```python
from build123d import *

# Parameters (mm, degrees)
F0_R      = 5
F1_DEPTH  = 15
F2_R      = 5
F4_DEPTH  = 15
F3_R      = 2.6
F5_DEPTH  = 25
F6_R      = 1.5
F7_DEPTH  = 10
F8_R      = 3.1
F9_DEPTH  = 1.5
F10_R     = 1.425
F11_DEPTH = 25
F12_R     = 2
F13_DEPTH = 1.5


with BuildPart() as f1:
    # F0 (on Front) → F1 (new body)
    with BuildSketch(Plane.XZ):
        Circle(F0_R)
    extrude(amount=F1_DEPTH)

    # F2 (on Top) → F4 (join)
    with BuildSketch(Plane.XY):
        with Locations((0, -9.121813)):
            Circle(F2_R)
    extrude(amount=F4_DEPTH)

    # F3 (on Front) → F5 (cut)
    with BuildSketch(Plane.XZ):
        Circle(F3_R)
    extrude(amount=F5_DEPTH, mode=Mode.SUBTRACT)

    # F6 (on face) → F7 (cut)
    with BuildSketch(Plane.XY.offset(15)):
        with Locations((0, -9.121813)):
            Circle(F6_R)
    extrude(amount=-F7_DEPTH, mode=Mode.SUBTRACT)

    # F8 (on face) → F9 (cut)
    with BuildSketch(Plane.XY.offset(15)):
        with Locations((0, -9.121813)):
            Circle(F8_R)
    extrude(amount=-F9_DEPTH, mode=Mode.SUBTRACT)

    # F10 (on Right) → F11 (cut)
    with BuildSketch(Plane.YZ):
        with Locations((-8.868461, 9.550918)):
            Circle(F10_R)
    extrude(amount=F11_DEPTH, mode=Mode.SUBTRACT)

    # F12 (on face) → F13 (cut)
    with BuildSketch(Plane.XY.offset(13.5)):
        with Locations((0, -9.121813)):
            Circle(F12_R)
    extrude(amount=-F13_DEPTH, mode=Mode.SUBTRACT)


solid = f1.part
```
Input: part model. Units: mm. Frame: model coordinates. A direction names the side the tool comes from. Round coordinates to 2 decimals unless told otherwise and drop trailing zeros. Loops run counter-clockwise (first coordinate to the right, second up) from the corner with the lowest first, then second, coordinate; pieces in that order, holes last. Notation, with made-up numbers: (28, -7.5) -> (33, -7.5) arc R4 cw to (33, -2.5) -> close; hole circle Ø4 at (-39.75, 48.5). An arc over 180 degrees is marked (long way). Use one line per item in the form item = value. Start each with the question number.
Item 1: Material intervals for L1, parallel to X at y = -8, z = 0; L2, parallel to Y at x = 0, z = 14.45; L3, parallel to Z at x = 0, y = -11.5, sorted ascending. Write a range as from..to.
Item 2: Section query A-A on z = 0.25. Return the cut outline in (x, y), then the cut area to 3 significant figures.
Item 3: Section query D-D on z = 10. Return the cut outline in (x, y).
Item 4: Mould query, pull axis Y, two halves, no side actions, for faces 1 (the face through (0, -9, 5)), 2 (the face through (2, 0, -2)), 3 (the face through (2, -15, -2)). Classes: pulls with the +Y half, pulls with the -Y half, needs draft (parallel to the pull), parting line crosses it, or undercut.
Item 5: Contact query for flat-ended pins moving along their axis: pin 1 Ø5 at (x, y) = (0, -12) entering from +Z; pin 2 Ø2.5 at (x, y) = (0.5, -9) entering from +Z; pin 3 Ø2 at (x, y) = (-1, -9.5) entering from +Z; pin 4 Ø3 at (x, z) = (-1, 11.5) entering from +Y. Output: stop coordinate, or through.
Item 6: Set-up query: faces 4 (the face through (-0.26, -7.14, 12.76)), 5 (the face through (-1.08, -7.4, -4.88)), 6 (the face through (3.02, -7.51, 9.98)), 7 (the face through (3.3, -9.1, 15)). Return all of +Z, -Z, +X, -X, +Y, -Y with unobstructed straight access to the full face (end or side cutting, diameter ignored); none if empty.
Item 7: Section query C-C on y = -11.75. Return the cut outline in (x, z), then the cut area to 3 significant figures.
Ans:
q1.L1 = -5..-2.6, 2.6..5
q1.L2 = -14.12..-12.22, -6.02..-4.12
q1.L3 = -5..-2.6, 2.6..13.5
q2.outline = (-4.99, -15) -> (-2.59, -15) -> (-2.59, 0) -> (-4.99, 0) -> (-4.99, -8.87) arc R5 ccw to (-4.99, -9.37) -> close; (2.59, -15) -> (4.99, -15) -> (4.99, -9.37) arc R5 ccw to (4.99, -8.87) -> (4.99, 0) -> (2.59, 0) -> close
q2.area = 72.2 mm^2
q3.outline = (0, -7.62) -> (0, -7.52) -> (4.74, -7.52) arc R5 ccw (long way) to (4.88, -10.22) -> (1.02, -10.22) arc R1.5 cw (long way) to start
q4.face_1 = undercut
q4.face_2 = pulls with the +Y half
q4.face_3 = pulls with the -Y half
q5.pin_1 = 15
q5.pin_2 = 12
q5.pin_3 = 13.5
q5.pin_4 = -4.12
q6.face_4 = +Z
q6.face_5 = none
q6.face_6 = +X
q6.face_7 = +Z, +X, -X, +Y, -Y
q7.outline = (-4.25, 2.63) arc R5 ccw (long way) to (4.25, 2.63) -> (4.25, 15) -> (1.64, 15) -> (1.64, 13.5) -> (-1.64, 13.5) -> (-1.64, 15) -> (-4.25, 15) -> close; hole circle Ø5.2 at (0, 0)
q7.area = 143 mm^2
